The listing builds one solid part. Answer for the finished solid, in the listing's coordinates (mm). A direction names the side the tool comes from. Round coordinates to 2 decimals unless told otherwise and drop trailing zeros. Write each loop counter-clockwise with the first axis right and the second up, starting at its lowest first coordinate (ties: lowest second). Pieces come first, ordered by that corner, then holes. Notation, with made-up numbers: (-11.75, -24.75) - (44.25, -24.75) arc R14 cw to (44.25, -5.75) - close; hole circle Ø5 at (87.25, -25.75). An arc over 180 degrees is marked (long way). Use a Markdown table: item, result. Add a question column.
1) Each of these flat-tipped pins is pushed along its axis until it touches: P1, Ø0.9, axis at x = 1.5, z = 10, coming from the -Y side; P2, Ø1, axis at x = 2, y = 4.5, coming from the -Z side; P3, Ø7, axis at x = 5.75, z = 7.25, coming from the +Y side; P4, Ø1.2, axis at x = 12, z = 4.5, coming from the -Y side. Where does it stop, or does it pass through?
2) A cutting plane is placed at C-C (y = 3). Give the vertices of the cut face in (x, z).
3) A cutting plane is placed at D-D (x = 5.75). Give the vertices of the cut face in (y, z).
4) A cutting plane is placed at A-A (y = 6.5). Give the vertices of the cut face in (x, z).
5) Determine the mould class of faces 1 (the flat face through (12.3, 0, 13.5)), 2 (the flat face through (13, 9, 7)), 3 (the flat face through (11.5, 8, 7)) for opening direction X: +X half, -X half, draft (parallel to the pull), parting line (faces both ways), or undercut.
6) A tool of negligible diameter and unlimited length cuts with its end or side. For faces 4 (the flat face through (0, 8, 7)), 5 (the flat face through (2.9, 15, 5.5)), 6 (the flat face through (-1, 2, 2)), from which of +Z, -Z, +X, -X, +Y, -Y can it reach the whole face along a straight path? Write none if from no direction.
7) A cutting plane is placed at B-B (z = 7.25). Give the vertices of the cut face in (x, y), then the cut area to 3 significant figures.
8) Find the intervals of material crossed by probe 1 along X at (y, z) = (12.5, 12.25); probe 2 along X at (y, z) = (13.2, 7.25); probe 3 along X at (y, z) = (14, 7.25), in increasing order. Write a range as from..to.
```python
from build123d import *

# Parameters (mm, degrees)
BOSS_EXTRUDE1_DEPTH = 14.5
CUT_EXTRUDE1_REACH  = 27.407
SKETCH2_W           = 4.25
SKETCH2_H           = 4
FILLET1_R           = 0.5
SKETCH3_R           = 3
CUT_EXTRUDE2_DEPTH  = 3


with BuildPart() as part:
    # Sketch1 → Boss-Extrude1 (new body)
    with BuildSketch(Plane.XY):
        with BuildLine():
            Line((0, 0), (-1.5, 0))
            Line((-1.5, 0), (-1.5, 14))
            ThreePointArc((-1.5, 14), (-1.207106781, 14.707106781), (-0.5, 15))
            Line((-0.5, 15), (12, 15))
            ThreePointArc((12, 15), (12.707106781, 14.707106781), (13, 14))
            Line((13, 14), (13, 0))
            Line((13, 0), (11.5, 0))
            Line((11.5, 0), (11.5, 13.5))
            Line((11.5, 13.5), (9.75, 13.5))
            Line((9.75, 13.5), (9.75, 12))
            Line((9.75, 12), (1.75, 12))
            Line((1.75, 12), (1.75, 13.5))
            Line((1.75, 13.5), (0, 13.5))
            Line((0, 13.5), (0, 0))
        make_face()
    extrude(amount=BOSS_EXTRUDE1_DEPTH)

    # Cut-Extrude1: up to this face of the body (flat: up to its plane)
    cut_extrude1_end = Plane(part.part.faces().sort_by_distance((-1.5, 7, 7.25))[0])
    # Sketch2 → Cut-Extrude1 (cut, up to the picked face)
    with BuildSketch(Plane(origin=(13, 0, 0), x_dir=(0, 0, -1), z_dir=(1, 0, 0)), mode=Mode.PRIVATE) as cut_extrude1_sk1:
        with Locations((-10.375, 2)):
            Rectangle(SKETCH2_W, SKETCH2_H)
    cut_extrude1_tool1 = split(extrude(cut_extrude1_sk1.sketch, amount=-CUT_EXTRUDE1_REACH, mode=Mode.PRIVATE), bisect_by=cut_extrude1_end, keep=Keep.BOTH, mode=Mode.PRIVATE)
    # Sketch2 → Cut-Extrude1 (cut, up to the picked face)
    with BuildSketch(Plane(origin=(13, 0, 0), x_dir=(0, 0, -1), z_dir=(1, 0, 0)), mode=Mode.PRIVATE) as cut_extrude1_sk2:
        with Locations((-4.125, 2)):
            Rectangle(SKETCH2_W, SKETCH2_H)
    cut_extrude1_tool2 = split(extrude(cut_extrude1_sk2.sketch, amount=-CUT_EXTRUDE1_REACH, mode=Mode.PRIVATE), bisect_by=cut_extrude1_end, keep=Keep.BOTH, mode=Mode.PRIVATE)
    add(cut_extrude1_tool1.solids().sort_by(Axis((13, 2, 10.375), (-1, 0, 0)))[0], mode=Mode.SUBTRACT)
    add(cut_extrude1_tool2.solids().sort_by(Axis((13, 2, 4.125), (-1, 0, 0)))[0], mode=Mode.SUBTRACT)

    # Fillet1
    fillet1_edges = [part.edges().sort_by_distance(p)[0] for p in [
        (-0.75, 0, 0),
        (12.25, 0, 0),
        (12.25, 0, 14.5),
        (-0.75, 0, 14.5),
        (-0.75, 0, 8.25),
        (12.25, 0, 8.25),
        (-0.75, 0, 12.5),
        (12.25, 0, 12.5),
        (-0.75, 0, 2),
        (12.25, 0, 2),
        (-0.75, 0, 6.25),
        (12.25, 0, 6.25),
    ]]
    fillet(fillet1_edges, radius=FILLET1_R)

    # Sketch3 → Cut-Extrude2 (cut)
    with BuildSketch(Plane(origin=(0, 15, 0), x_dir=(1, 0, 0), z_dir=(0, 1, 0))):
        with Locations(Location((5.75, -7.25, 0), (0, 0, 270))):
            Circle(SKETCH3_R)
    extrude(amount=-CUT_EXTRUDE2_DEPTH, mode=Mode.SUBTRACT)


solid = part.part
```
Entries:
| question | item | result |
|---|---|---|
| 1 | P1 | stops at y = 12 |
| 1 | P2 | passes through |
| 1 | P3 | stops at y = 15 |
| 1 | P4 | stops at y = 4 |
| 2 | outline | (-1.5, 0) - (0, 0) - (0, 2) - (-1.5, 2) - close; (-1.5, 6.25) - (0, 6.25) - (0, 8.25) - (-1.5, 8.25) - close; (-1.5, 12.5) - (0, 12.5) - (0, 14.5) - (-1.5, 14.5) - close; (11.5, 0) - (13, 0) - (13, 2) - (11.5, 2) - close; (11.5, 6.25) - (13, 6.25) - (13, 8.25) - (11.5, 8.25) - close; (11.5, 12.5) - (13, 12.5) - (13, 14.5) - (11.5, 14.5) - close |
| 3 | outline | (12, 0) - (15, 0) - (15, 4.25) - (12, 4.25) - close; (12, 10.25) - (15, 10.25) - (15, 14.5) - (12, 14.5) - close |
| 4 | outline | (-1.5, 0) - (0, 0) - (0, 14.5) - (-1.5, 14.5) - close; (11.5, 0) - (13, 0) - (13, 14.5) - (11.5, 14.5) - close |
| 5 | face 1 | draft |
| 5 | face 2 | +X half |
| 5 | face 3 | undercut |
| 6 | face 4 | +Z, -Z, -Y |
| 6 | face 5 | +Z, -Z, +X, -X, +Y |
| 6 | face 6 | +X, -X, -Y |
| 7 | outline | (-1.5, 0) - (0, 0) - (0, 13.5) - (1.75, 13.5) - (1.75, 12) - (2.75, 12) - (2.75, 15) - (-0.5, 15) arc R1 ccw to (-1.5, 14) - close; (8.75, 12) - (9.75, 12) - (9.75, 13.5) - (11.5, 13.5) - (11.5, 0) - (13, 0) - (13, 14) arc R1 ccw to (12, 15) - (8.75, 15) - close |
| 7 | area | 55.8 mm² |
| 8 | probe 1 | x = -1.5..0, 1.75..9.75, 11.5..13 |
| 8 | probe 2 | x = -1.5..0, 1.75..2.75, 8.75..9.75, 11.5..13 |
| 8 | probe 3 | x = -1.5..2.75, 8.75..13 |
